```python
from build123d import *

# Parameters (mm, degrees)
SKETCH1_R           = 40
BOSS_EXTRUDE1_DEPTH = 150
SKETCH2_R           = 20
BOSS_EXTRUDE2_DEPTH = 40
SKETCH3_W           = 40.516071082
SKETCH3_H           = 80
CUT_EXTRUDE1_DEPTH  = 50
SKETCH4_R           = 21.141799796
CUT_EXTRUDE2_DEPTH  = 10
FILLET1_R           = 40
FILLET2_R           = 5


with BuildPart() as part:
    # Sketch1 → Boss-Extrude1 (new body)
    with BuildSketch(Plane(origin=(0, 0, 0), x_dir=(1, 0, 0), z_dir=(0, 1, 0))):
        with Locations(Location((0, 0, 0), (0, 0, 270))):
            Circle(SKETCH1_R)
    extrude(amount=BOSS_EXTRUDE1_DEPTH)

    # Sketch2 → Boss-Extrude2 (add)
    with BuildSketch(Plane.XZ):
        with Locations(Location((0, 0, 0), (0, 0, 270))):
            Circle(SKETCH2_R)
    extrude(amount=BOSS_EXTRUDE2_DEPTH)

    # Sketch3 → Cut-Extrude1 (cut)
    with BuildSketch(Plane(origin=(0, 150, 0), x_dir=(1, 0, 0), z_dir=(0, 1, 0))):
        with Locations((20.258035541, 0)):
            Rectangle(SKETCH3_W, SKETCH3_H)
    extrude(amount=-CUT_EXTRUDE1_DEPTH, mode=Mode.SUBTRACT)

    # Sketch4 → Cut-Extrude2 (cut)
    with BuildSketch(Plane(origin=(0, 0, 0), x_dir=(0, 0, -1), z_dir=(1, 0, 0))):
        with Locations((0, 125.6230245)):
            Circle(SKETCH4_R)
    extrude(amount=-CUT_EXTRUDE2_DEPTH, mode=Mode.SUBTRACT)

    # Fillet1
    fillet1_edges = [part.edges().sort_by_distance(p)[0] for p in [
        (-40, 150, 0),
    ]]
    fillet(fillet1_edges, radius=FILLET1_R - 0.0001)  # a hair under: the kernel refuses the full size

    # Fillet2
    fillet2_edges = [part.edges().sort_by_distance(p)[0] for p in [
        (0, 0, -40),
    ]]
    fillet(fillet2_edges, radius=FILLET2_R)


solid = part.part
```
Could you check a few things on this model? Use its own coordinates, in mm. A direction names the side the tool comes from. Give positions to 0.01 mm unless a question says otherwise; leave off trailing zeros. Loops run counter-clockwise (first coordinate to the right, second up) from the corner with the lowest first, then second, coordinate; pieces in that order, holes last. Notation, with made-up numbers: (85, 10) - (136, 10) arc R25 ccw to (136, 35) - close; hole circle Ø9 at (61.5, 87). An arc over 180 degrees is marked (long way). Answer in a Markdown table with one row per item. Add a question column.
Q1. If we section it at B-B (y = 73.5): List the corners of the cut face in (x, z) for me, plus the area to 3 significant figures.
Q2. We'd pull the mould along Z, two halves only. Please class faces 1 (the face through (-4.93, 146.585, 2.752)), 2 (the face through (-39.05, 56.77, -8.67)), 3 (the face through (15, 100, -1)): +Z half, -Z half, draft (parallel to the pull), parting line (faces both ways), or undercut.
Q3. Please list where these lines run through material, in increasing order: L1, parallel to Y at x = 11, z = 26; L2, parallel to Y at x = -3, z = 0; L3, parallel to Y at x = -6.5, z = 0. Write a range as from..to.
Q4. If we section it at A-A (y = -26.5): List the corners of the cut face in (x, z) for me.
Q5. For pin 1 (10 mm diameter, centred on x = 24.5, y = 1.5, fed in from -Z); pin 2 (10 mm diameter, centred on y = 101, z = -14.5, fed in from -X); pin 3 (3 mm diameter, centred on y = 86, z = 22, fed in from +X), each with a flat end and sliding along its axis, tell me the tip position at first contact or that it passes through.
Q6. Which directions (+Z, -Z, +X, -X, +Y, -Y) give clear straight access to the entire face, cutting with the end or side of a thin tool? Please do faces 4 (the face through (0, 103, 1)), 5 (the face through (-10, 126, 0)), 6 (the face through (-15, 0, 15)).
The answers:
| question | item | result |
|---|---|---|
| 1 | outline | circle Ø80 at (0, 0) |
| 1 | area | 5,030 mm^2 |
| 2 | face 1 | undercut |
| 2 | face 2 | parting line |
| 2 | face 3 | draft |
| 3 | L1 | y = 0..100 |
| 3 | L2 | y = -40..104.48, 146.76..149.89 |
| 3 | L3 | y = -40..104.48, 146.76..149.47 |
| 4 | outline | circle Ø40 at (0, 0) |
| 5 | pin 1 | stops at z = -34.44 |
| 5 | pin 2 | stops at x = -38.86 |
| 5 | pin 3 | stops at x = 34.35 |
| 6 | face 4 | +Z, -Z, +X, +Y |
| 6 | face 5 | +X |
| 6 | face 6 | -Y |
